Autodesk Fusion 360 part; units mm, degrees
sketch "Sketch1" plane through (0, 0, 0) normal (0, 0, 1) x (1, 0, 0)
  line L0 (0, 0) -> (-70, 0)
  line L1 (-70, 0) -> (-70, 90)
  line L2 (-70, 90) -> (0, 90)
  line L3 (0, 90) -> (0, 0)
  line L4 (-70, 0) -> (0, 0)
  line L5 (0, 0) -> (0, 10)
  line L6 (0, 10) -> (-70, 10)
  line L7 (-70, 10) -> (-70, 0)
  line L8 (-70, 10) -> (-35, 10)
  line L9 (0, 10) -> (0, 32.5)
  line L10 (-35, 10) -> (-15, 10)
  line L11 (-15, 10) -> (-15, 37.5)
  line L12 (-15, 10) -> (-35, 10)
  line L13 (-35, 10) -> (-35, 37.5)
  line L14 (-35, 37.5) -> (-15, 37.5)
  line L15 (-15, 37.5) -> (-15, 10)
  ellipse E0 centre (-35, 37.5) end of major axis (-35, 10) minor radius 20
  line L16 (-35, 65) -> (-35, 10) construction
  line L17 (-55, 37.5) -> (-15, 37.5) construction
  line L18 (0, 10) -> (-10, 10)
  line L19 (-10, 10) -> (-60, 10)
  line L20 (-60, 10) -> (-60, 72.5)
  line L21 (-60, 72.5) -> (-10, 72.5)
  line L22 (-10, 72.5) -> (-10, 10)
  line L23 (0, 10) -> (-70, 10)
  line L24 (-70, 10) -> (-70, 2.5)
  line L25 (-70, 2.5) -> (0, 2.5)
  line L26 (0, 2.5) -> (0, 10)
  line L27 (0, 2.5) -> (-70, 2.5)
  line L28 (-70, 2.5) -> (-70, -7.5)
  line L29 (-70, -7.5) -> (0, -7.5)
  line L30 (0, -7.5) -> (0, 2.5)
  line L31 (-10, 10) -> (-60, 10)
  line L32 (-60, 10) -> (-60, 2.5)
  line L33 (-60, 2.5) -> (-10, 2.5)
  line L34 (-10, 2.5) -> (-10, 10)
  line L35 (0, -7.5) -> (5, -7.5)
  line L36 (5, -7.5) -> (5, -12.5)
  line L37 (5, -12.5) -> (0, -12.5)
  line L38 (0, -12.5) -> (0, -7.5)
  line L39 (5, -12.5) -> (-75, -12.5)
  line L40 (-75, -12.5) -> (-75, 95)
  line L41 (-75, 95) -> (5, 95)
  line L42 (5, 95) -> (5, -12.5)
  dimension "d1" = 70
  dimension "d2" = 90
  dimension "d3" = 10
  dimension "d4" = 35
  dimension "d5" = 22.5
  dimension "d6" = 20
  dimension "d7" = 27.5
  dimension "d8" = 27.5
  dimension "d11" = 10
  dimension "d12" = 50
  dimension "d13" = 62.5
  dimension "d14" = 70
  dimension "d15" = 7.5
  dimension "d16" = 70
  dimension "d17" = 10
  dimension "d20" = 50
  dimension "d21" = 7.5
  dimension "d22" = 5
  dimension "d23" = 5
  dimension "d24" = 80
  dimension "d25" = 107.5
extrude "Extrude1" add sketch "Sketch1" along normal blind 27 contours L0 L1 L3 L4 L5 L7 L25 L27 L28 L30 L33 | L3 L5 L6 L18 L23 L25 L26 L27 L34 | L1 L6 L7 L8 L23 L24 L25 L27 L32 | L1 L2 L3 L6 L8 L9 L18 L20 L21 L22 L23 | L6 L8 L10 L12 L19 L23 L25 L27 L31 L32 L33 L34 | L6 L8 L11 L15 E0 L19 L20 L21 L22 L23 L31 | L6 L10 L11 L12 L15 E0 L19 L23 L31
extrude "Extrude2" add sketch "Sketch1" along normal blind 27 contours L0 L4 L28 L29 L30
sketch "Sketch2" plane through (0, 0, 27) normal (0, 0, 1) x (-1, 0, 0)
  ellipse E0 centre (35, -37.5) end of major axis (35, -10) minor radius 20
  line L0 (70, -90) -> (70, 7.5)
  line L1 (70, 7.5) -> (0, 7.5)
  line L2 (0, 7.5) -> (0, -90)
  line L3 (0, -90) -> (70, -90)
  ellipse E1 centre (35, -37.5) end of major axis (35, -10) minor radius 20
  line L4 (35, -65) -> (35, -10) construction
  line L5 (55, -37.5) -> (15, -37.5) construction
loft "Loft1" cut profiles "Sketch2", "Sketch1" section 1 contours E0 E1 section 2 contours L6 L8 L10 L12 L19 L23 L25 L27 L31 L32 L33 L34 | L6 L8 L11 L15 E0 L19 L20 L21 L22 L23 L31 | L6 L10 L11 L12 L15 E0 L19 L23 L31
extrude "Extrude3" add sketch "Sketch1" along normal blind 27
sketch "Sketch3" plane through (0, 0, 0) normal (0, 0, -1) x (1, 0, 0)
  line L0 (-75, -95) -> (5, -95)
  line L1 (5, -95) -> (5, 12.5)
  line L2 (5, 12.5) -> (-75, 12.5)
  line L3 (-75, 12.5) -> (-75, -95)
  line L4 (-60, -72.5) -> (-60, -2.5)
  line L5 (-60, -2.5) -> (-10, -2.5)
  line L6 (-10, -2.5) -> (-10, -72.5)
  line L7 (-10, -72.5) -> (-60, -72.5)
sketch "Sketch4" plane through (0, 0, 0) normal (0, 0, -1) x (1, 0, 0)
  line L0 (-75, -95) -> (5, -95)
  line L1 (5, -95) -> (5, 12.5)
  line L2 (5, 12.5) -> (-75, 12.5)
  line L3 (-75, 12.5) -> (-75, -95)
  line L4 (-60, -72.5) -> (-60, -2.5)
  line L5 (-60, -2.5) -> (-10, -2.5)
  line L6 (-10, -2.5) -> (-10, -72.5)
  line L7 (-10, -72.5) -> (-60, -72.5)
  line L8 (-75, 12.5) -> (-72.5, 12.5)
  line L9 (-72.5, 12.5) -> (-72.5, 10)
  line L10 (-72.5, 10) -> (-75, 10)
  line L11 (-75, 10) -> (-75, 12.5)
  line L12 (-60, -2.5) -> (-62.5, -2.5)
  line L13 (-62.5, -2.5) -> (-62.5, 0)
  line L14 (-62.5, 0) -> (-60, 0)
  line L15 (-60, 0) -> (-60, -2.5)
  line L16 (5, 12.5) -> (3.2245, 12.5)
  line L17 (3.2245, 12.5) -> (3.2245, 10)
  line L18 (3.2245, 10) -> (5, 10)
  line L19 (5, 10) -> (5, 12.5)
  line L20 (-62.5, 0) -> (-7.5, 0)
  line L21 (-7.5, 0) -> (-7.5, -75)
  line L22 (-7.5, -75) -> (-62.5, -75)
  line L23 (-62.5, -75) -> (-62.5, 0)
  line L24 (5, -95) -> (2.5, -95)
  line L25 (2.5, -95) -> (2.5, -92.5)
  line L26 (2.5, -92.5) -> (5, -92.5)
  line L27 (5, -92.5) -> (5, -95)
  line L28 (-72.5, 10) -> (2.5, 10)
  line L29 (2.5, 10) -> (2.5, -92.5)
  line L30 (2.5, -92.5) -> (-72.5, -92.5)
  line L31 (-72.5, -92.5) -> (-72.5, 10)
  line L32 (-75, 12.5) -> (5, 12.5)
  line L33 (5, 12.5) -> (5, -95)
  line L34 (5, -95) -> (-75, -95)
  line L35 (-75, -95) -> (-75, 12.5)
  line L36 (-62.5, -75) -> (-55.5, -75)
  line L37 (-7.5, -75) -> (-14.5, -75)
  line L38 (-55.5, -75) -> (-55.5, -72.5)
  line L39 (-14.5, -75) -> (-55.5, -75)
  line L40 (-55.5, -75) -> (-55.5, -72.5)
  line L41 (-55.5, -72.5) -> (-14.5, -72.5)
  line L42 (-14.5, -72.5) -> (-14.5, -75)
  line L43 (-14.5, -75) -> (-55.5, -75)
  line L44 (-55.5, -75) -> (-55.5, -62.3242)
  line L45 (-55.5, -62.3242) -> (-14.5, -62.3242)
  line L46 (-14.5, -62.3242) -> (-14.5, -75)
  line L47 (-30, -95) -> (-40, -95)
  line L48 (-40, -95) -> (-40, -92.5)
  line L49 (-40, -92.5) -> (-30, -92.5)
  line L50 (-30, -92.5) -> (-30, -95)
  dimension "d30" = 2.5
  dimension "d31" = 2.5
  dimension "d32" = 2.5
  dimension "d33" = 2.5
  dimension "d34" = 2.5
  dimension "d35" = 55
  dimension "d36" = 75
  dimension "d37" = 2.5
  dimension "d38" = 2.5
  dimension "d39" = 7
  dimension "d40" = 7
  dimension "d41" = 10
extrude "Extrude4" cut sketch "Sketch4" against normal blind 10 contours L7 L41 L44 L45 L46 | L7 L22 L38 L39 L40 L41 L42 L43 L44 L46
fillet "Fillet1" radius 10 2 edges at (-14.5, 70.9614, 10) (-55.5, 70.9614, 10)
extrude "Extrude5" cut sketch "Sketch4" against normal blind 10 contours L28 L29 L30 L31 L49
fillet "Fillet2" radius 5 9 edges at (2.5, 41.25, 10) (-35, 92.5, 10) (-7.5, 37.5, 10) (-62.5, 37.5, 10) (-72.5, 41.25, 10) (-35, -10, 10) (-35, 0, 10) (-54, 75, 10) (-16, 75, 10)
extrude "Extrude6" cut sketch "Sketch4" against normal blind 5 contours L0 L30 L34 L47 L48 L49 L50
fillet "Fillet3" radius 5 2 edges at (-40, 93.75, 5) (-30, 93.75, 5)
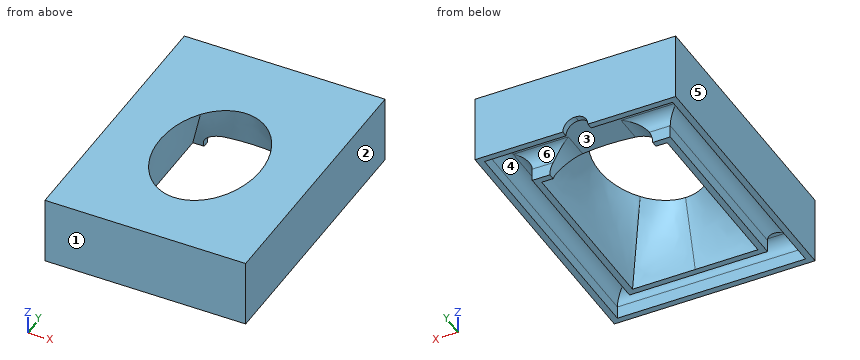
Verification items for the finished model (mm, model axes). Face numbers are marked on the shaded views. A direction names the side the tool comes from. Coordinates: 2 decimals unless noted, no trailing zeros. One line per item, written item: value. Start each with the question number.
Item 1: Access from +Z, -Z, +X, -X, +Y, -Y to the whole of each face (thin tool, end or side, straight path). Record for the marked faces 5 and 6.
Item 2: Scan lines: probe 1 along Y at (x, z) = (-41.5, 3.5); probe 2 along X at (y, z) = (24, 2.25); probe 3 along Y at (x, z) = (-25, 6). Record each from-to range of solid material in increasing order.
Item 3: Mould release check, pull along X, two halves, no side actions. Record for the marked faces 1, 2, 3 and 4: released by +X, released by -X, zero draft, split by the parting line, or undercut.
Item 4: Gauge pin test, flat ends, axial feed: pin 1 (2 mm diameter, centred on x = -57, y = 6, fed in from -Z); pin 2 (10 mm diameter, centred on x = -50.5, y = -1.5, fed in from -Z); pin 3 (5 mm diameter, centred on x = -24, y = 13, fed in from -Z). Record the tip position at first contact, or that the pin passes through.
Conclusion:
1. face 5: +Z, -Z, -X, +Y, -Y
1. face 6: -Z
2. probe 1: y = -12.5 to -10, 0 to 3.55, 92.5 to 95
2. probe 2: x = -75 to -72.5, -62.5 to -59.5, -10.5 to -7.5, 2.5 to 5
2. probe 3: y = -12.5 to -9.9, -0.1 to 4.52, 92.4 to 95
3. face 1: zero draft
3. face 2: released by +X
3. face 3: undercut
3. face 4: undercut
4. pin 1: stops at z = 4.6
4. pin 2: stops at z = 0
4. pin 3: stops at z = 19.66
